Check sheet for the modelled part. Datum: model origin and axes. Units: mm. Face numbers are marked on the shaded views. A direction names the side the tool comes from. Round coordinates to 2 decimals unless told otherwise and drop trailing zeros. Loops run counter-clockwise (first coordinate to the right, second up) from the corner with the lowest first, then second, coordinate; pieces in that order, holes last. Notation, with made-up numbers: (-29, 76) - (13, 76) arc R29 cw to (13, 103) - close; hole circle Ø6 at (75.25, -1). An arc over 180 degrees is marked (long way). Put each result on its own line as item: value.
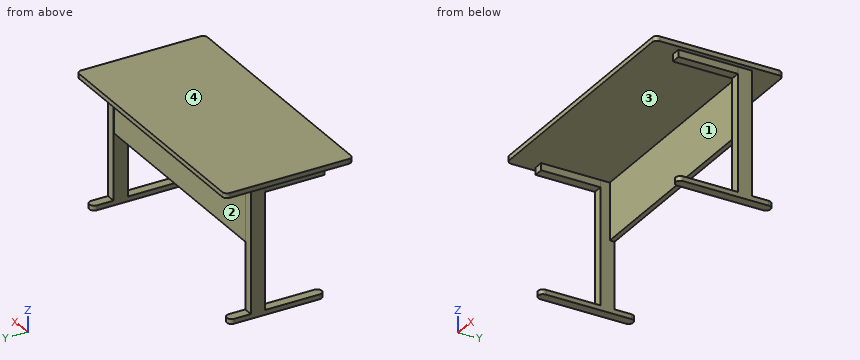
```python
from build123d import *

# Parameters (mm, degrees)
F1_DEPTH = 25.4
F2_W     = 50.8
F2_H     = 317.5
F3_DEPTH = 38.1
F4_W     = 50.8
F4_H     = 76.2
F5_DEPTH = 660.4
F6_W     = 1195.401192
F6_H     = 25.4
F7_DEPTH = 304.8
F9_DEPTH = 25.4


with BuildPart() as f1:
    # F0 (on Top) → F1 (new body)
    with BuildSketch(Plane.XY):
        with BuildLine():
            Line((0, -342.9), (648.97, -342.9))
            ThreePointArc((648.97, -342.9), (666.930512, -335.460512), (674.37, -317.5))
            Line((674.37, -317.5), (674.37, 317.5))
            ThreePointArc((674.37, 317.5), (666.930512, 335.460512), (648.97, 342.9))
            Line((648.97, 342.9), (0, 342.9))
            Line((0, 342.9), (0, -342.9))
        make_face()
        with BuildLine():
            Line((-648.97, -342.9), (0, -342.9))
            Line((0, -342.9), (0, 342.9))
            Line((0, 342.9), (-648.97, 342.9))
            ThreePointArc((-648.97, 342.9), (-666.930512, 335.460512), (-674.37, 317.5))
            Line((-674.37, 317.5), (-674.37, -317.5))
            ThreePointArc((-674.37, -317.5), (-666.930512, -335.460512), (-648.97, -342.9))
        make_face()
    extrude(amount=F1_DEPTH)

    # F2 (on Top) → F3 (join)
    with BuildSketch(Plane.XY):
        with Locations((-623.57, -44.45)):
            Rectangle(F2_W, F2_H)
        with Locations((623.57, -44.45)):
            Rectangle(F2_W, F2_H)
    extrude(amount=-F3_DEPTH)

    # F4 (on face) → F5 (join)
    with BuildSketch(Plane.XY):
        with Locations((-623.534083, 152.223289)):
            Rectangle(F4_W, F4_H)
        with Locations((623.534083, 152.223289)):
            Rectangle(F4_W, F4_H)
    extrude(amount=-F5_DEPTH)

    # F6 (on Top) → F7 (join)
    with BuildSketch(Plane.XY):
        with Locations((0, 176.231914)):
            Rectangle(F6_W, F6_H)
    extrude(amount=-F7_DEPTH)

    # F8 (on face) → F9 (join)
    with BuildSketch(Plane(origin=(0, 0, -660.4), x_dir=(1, 0, 0), z_dir=(0, 0, -1))):
        with BuildLine():
            ThreePointArc((-623.534083, 203.559189), (-641.494596, 196.119702), (-648.934083, 178.159189))
            Line((-648.934083, 178.159189), (-648.934083, -279.040811))
            ThreePointArc((-648.934083, -279.040811), (-641.494596, -297.001323), (-623.534083, -304.440811))
            ThreePointArc((-623.534083, -304.440811), (-605.573571, -297.001323), (-598.134083, -279.040811))
            Line((-598.134083, -279.040811), (-598.134083, 178.159189))
            ThreePointArc((-598.134083, 178.159189), (-605.573571, 196.119702), (-623.534083, 203.559189))
        make_face()
        with BuildLine():
            ThreePointArc((623.534083, 203.559189), (605.573571, 196.119702), (598.134083, 178.159189))
            Line((598.134083, 178.159189), (598.134083, -279.040811))
            ThreePointArc((598.134083, -279.040811), (605.573571, -297.001323), (623.534083, -304.440811))
            ThreePointArc((623.534083, -304.440811), (641.494596, -297.001323), (648.934083, -279.040811))
            Line((648.934083, -279.040811), (648.934083, 178.159189))
            ThreePointArc((648.934083, 178.159189), (641.494596, 196.119702), (623.534083, 203.559189))
        make_face()
    extrude(amount=F9_DEPTH)


solid = f1.part
```
Item 1: Release check for a two-part mould opening along X. For the marked faces 3 and 4 record: +X half, -X half, draft (parallel to the pull), parting line (faces both ways), or undercut.
Filled sheet:
face 3: undercut
face 4: draft
Item 2: Go/stop test with flat-tipped pins: pin 1 (1 mm diameter, centred on x = 256, z = -81.5, fed in from +Y); pin 2 (10 mm diameter, centred on x = 318, z = -103.5, fed in from -Y); pin 3 (11.5 mm diameter, centred on x = -612, z = -21.5, fed in from -Y). Record where each tip stops, or that it passes through.
Filled sheet:
pin 1: y = 188.93
pin 2: y = 163.53
pin 3: y = -203.2
Item 3: Section check B-B on y = -160. Enter the section's corners in (x, z).
Filled sheet:
outline: (-674.37, 0) - (-648.97, 0) - (-648.97, -38.1) - (-598.17, -38.1) - (-598.17, 0) - (598.17, 0) - (598.17, -38.1) - (648.97, -38.1) - (648.97, 0) - (674.37, 0) - (674.37, 25.4) - (-674.37, 25.4) - close; (-648.93, -685.8) - (-598.13, -685.8) - (-598.13, -660.4) - (-648.93, -660.4) - close; (598.13, -685.8) - (648.93, -685.8) - (648.93, -660.4) - (598.13, -660.4) - close
Item 4: Tool access check on the marked faces 1 and 2. Record the directions out of +Z, -Z, +X, -X, +Y, -Y that give a thin tool (end or side, any length) a straight path to the whole face; none if there is none.
Filled sheet:
face 1: -Z, -Y
face 2: -Z, +Y
Item 5: Section check D-D on x = -190.5. Enter the section's corners in (y, z).
Filled sheet:
outline: (-342.9, 0) - (163.53, 0) - (163.53, -304.8) - (188.93, -304.8) - (188.93, 0) - (342.9, 0) - (342.9, 25.4) - (-342.9, 25.4) - close
Item 6: Section check A-A on z = -169.5. Enter the section's corners in (x, y), then the cut area to 3 significant figures.
Filled sheet:
outline: (-648.93, 114.12) - (-598.13, 114.12) - (-598.13, 190.32) - (-648.93, 190.32) - close; (-597.7, 163.53) - (597.7, 163.53) - (597.7, 188.93) - (-597.7, 188.93) - close; (598.13, 114.12) - (648.93, 114.12) - (648.93, 190.32) - (598.13, 190.32) - close
area: 38,100 mm²
Item 7: Section check C-C on z = -595. Enter the section's corners in (x, y), then the cut area to 3 significant figures.
Filled sheet:
outline: (-648.93, 114.12) - (-598.13, 114.12) - (-598.13, 190.32) - (-648.93, 190.32) - close; (598.13, 114.12) - (648.93, 114.12) - (648.93, 190.32) - (598.13, 190.32) - close
area: 7,740 mm²
Item 8: Thickness scan on line 1 (X direction, y = 146, z = -306); line 2 (Y direction, x = -32, z = -240.5); line 3 (Z direction, x = -11.5, y = -130). Record the ranges inside material, lowest first. Write a range as from..to.
Filled sheet:
line 1: -648.93..-598.13, 598.13..648.93
line 2: 163.53..188.93
line 3: 0..25.4
